Source: CAD feature listing. Evaluate the final solid. Frame: model axes, mm. A direction names the side the tool comes from. Give positions to 0.01 mm unless a question says otherwise; leave off trailing zeros. Write each loop counter-clockwise with the first axis right and the second up, starting at its lowest first coordinate (ties: lowest second). Pieces come first, ordered by that corner, then holes. Notation, with made-up numbers: (-14, -39) - (3, -39) arc R8 ccw to (3, -24) - close; hole circle Ø9 at (72.25, 86). An arc over 180 degrees is marked (long way). One line per question, with ' | ' between items. Start each with the question number.
(1) Section D-D, the plane y = -28.5. Return loops of the section in (x, z) (3 decimals).
(2) Section A-A, the plane z = -1. Return loops of the section in (x, y).
(3) Ray query, line 1 (X direction, y = -0.5, z = -2); line 2 (Z direction, x = 14, y = -13) (3 decimals); line 3 (X direction, y = -35.5, z = 2.5). Return the intervals inside material, ascending. Write a range as [from, to].
(4) Pin query (flat end, axial travel): pin 1 (4 mm diameter, centred on x = 9.5, z = 4, fed in from -Y); pin 2 (1.5 mm diameter, centred on y = 16, z = -1, fed in from -X); pin 3 (2.5 mm diameter, centred on y = -31.5, z = 1, fed in from +X); pin 4 (1.5 mm diameter, centred on x = -4, z = 5, fed in from -Y). Return the tip coordinate at first contact, or that it passes through.
(5) Access query for faces 1 (the cylindrical face through (2.3, -19.8, -1.6)), 2 (the flat face through (2, 23.298, -2)), 3 (the flat face through (2.853, 2, -2)), 4 (the cylindrical face through (10.4, -21.15, 1.57)). Directions: +Z, -Z, +X, -X, +Y, -Y. A direction counts if a zero-diameter tool reaches every point of the face in a straight line with its end or side. Return the directions, or none.
(6) Section B-B, the plane y = 2. Return loops of the section in (x, z) (3 decimals).
(7) Section C-C, the plane x = 0. Return loops of the section in (y, z) (3 decimals).
(8) Draft query along Z for faces 5 (the flat face through (0, -19, 6.35)), 6 (the cylindrical face through (-0.27, 30.78, 1.57)), 7 (the flat face through (-1.651, 2, -1)). Return one class per face: +Z half, -Z half, draft (parallel to the pull), parting line (faces both ways), or undercut.
```python
from build123d import *

# Parameters (mm, degrees)
BOSS_EXTRUDE1_DEPTH = 3.175
BOSS_EXTRUDE2_DEPTH = 3.175
SKETCH3_W           = 6.236959702
SKETCH3_H           = 41.352711554
BOSS_EXTRUDE3_DEPTH = 3.175
SKETCH4_R           = 1.27
BOSS_EXTRUDE4_DEPTH = 3.175
BOSS_EXTRUDE5_REACH = 20.766
SKETCH6_W           = 0.889
SKETCH6_H           = 43.066281197
CUT_EXTRUDE1_REACH  = 11.525


with BuildPart() as part:
    # Sketch1 → Boss-Extrude1 (new body)
    with BuildSketch(Plane.XY):
        with BuildLine():
            Line((-17.114253333, -23.707583903), (-17.114253333, 23.707583903))
            ThreePointArc((-17.114253333, 23.707583903), (0, 30.782200079), (17.114253333, 23.707583903))
            Line((17.114253333, 23.707583903), (17.114253333, -23.707583903))
            ThreePointArc((17.114253333, -23.707583903), (0, -19.732802645), (-17.114253333, -23.707583903))
        make_face()
    extrude(amount=BOSS_EXTRUDE1_DEPTH)

    # Sketch2 → Boss-Extrude2 (add)
    with BuildSketch(Plane(origin=(0, 0, 0), x_dir=(-1, 0, 0), z_dir=(0, 0, -1))):
        with BuildLine():
            Line((-1.65128862, -19.767928257), (-1.65128862, 22.268343179))
            Line((-1.65128862, 22.268343179), (-1.65128862, 23.29835294))
            Line((-1.65128862, 23.29835294), (-2.853426735, 23.29835294))
            Line((-2.853426735, 23.29835294), (-2.853426735, -19.837781624))
            ThreePointArc((-2.853426735, -19.837781624), (-2.25262846, -19.798194915), (-1.65128862, -19.767928257))
        make_face()
        with BuildLine():
            Line((1.65128862, 23.29835294), (1.65128862, 22.268343179))
            Line((1.65128862, 22.268343179), (1.65128862, -19.767928257))
            ThreePointArc((1.65128862, -19.767928257), (2.25262846, -19.798194915), (2.853426735, -19.837781624))
            Line((2.853426735, -19.837781624), (2.853426735, 23.29835294))
            Line((2.853426735, 23.29835294), (1.65128862, 23.29835294))
        make_face()
    extrude(amount=BOSS_EXTRUDE2_DEPTH)

    # Sketch3 → Boss-Extrude3 (add)
    with BuildSketch(Plane.XY.offset(3.175)):
        with Locations((0, -20.33746726)):
            Rectangle(SKETCH3_W, SKETCH3_H)
    extrude(amount=-BOSS_EXTRUDE3_DEPTH)

    # Sketch4 → Boss-Extrude4 (add)
    with BuildSketch(Plane.XY.offset(3.175)):
        with Locations((0, -19.105823038)):
            Circle(SKETCH4_R)
    extrude(amount=BOSS_EXTRUDE4_DEPTH)

    # Sketch6 → Boss-Extrude5 (add, up to next)
    with BuildSketch(Plane.ZY.offset(-1.65128862), mode=Mode.PRIVATE) as boss_extrude5_sk1:
        with Locations((-2.7305, 1.765212341)):
            Rectangle(SKETCH6_W, SKETCH6_H)
    boss_extrude5_tool1 = extrude(boss_extrude5_sk1.sketch, amount=BOSS_EXTRUDE5_REACH, mode=Mode.PRIVATE) - part.part
    add(boss_extrude5_tool1.solids().sort_by_distance((1.651289, 1.765212, -2.7305))[0])

    # Sketch8 → Cut-Extrude1 (cut, up to next)
    with BuildSketch(Plane(origin=(0, 0, -3.175), x_dir=(-1, 0, 0), z_dir=(0, 0, -1)), mode=Mode.PRIVATE) as cut_extrude1_sk1:
        Polygon((0, 23.29835294), (-1.016, 23.29835294), (-1.016, -19.767928257), (1.016, -19.767928257), (1.016, 23.29835294), align=None)
    cut_extrude1_tool1 = extrude(cut_extrude1_sk1.sketch, amount=-CUT_EXTRUDE1_REACH, mode=Mode.PRIVATE) & part.part
    add(cut_extrude1_tool1.solids().sort_by_distance((0, 1.765212, -3.175))[0], mode=Mode.SUBTRACT)


solid = part.part
```
Check sheet entries:
1) outline: (-3.118, 0) - (3.118, 0) - (3.118, 3.175) - (-3.118, 3.175) - close
2) outline: (-2.85, -19.84) arc R38.83 cw to (-1.65, -19.77) - (-1.65, 23.3) - (-2.85, 23.3) - close; (1.65, -19.77) arc R38.83 cw to (2.85, -19.84) - (2.85, 23.3) - (1.65, 23.3) - close
3) line 1: [-2.85, -1.65], [1.65, 2.85] | line 2: [0, 3.175] | line 3: [-3.12, 3.12]
4) pin 1: y = -21.42 | pin 2: x = -2.85 | pin 3: x = 3.12 | pin 4: through
5) face 1: -Z, -Y | face 2: -Z, +X, -X, +Y | face 3: -Z, +X, +Y, -Y | face 4: +Z, -Z, -Y
6) outline: (-17.114, 0) - (-2.853, 0) - (-2.853, -3.175) - (-1.016, -3.175) - (-1.016, -2.286) - (-1.651, -2.286) - (-1.651, 0) - (1.651, 0) - (1.651, -2.286) - (1.016, -2.286) - (1.016, -3.175) - (2.853, -3.175) - (2.853, 0) - (17.114, 0) - (17.114, 3.175) - (-17.114, 3.175) - close
7) outline: (-41.014, 0) - (30.782, 0) - (30.782, 3.175) - (-17.836, 3.175) - (-17.836, 6.35) - (-20.376, 6.35) - (-20.376, 3.175) - (-41.014, 3.175) - close
8) face 5: +Z half | face 6: draft | face 7: undercut
